```python
from build123d import *

# Parameters (mm, degrees)
F1_W     = 59.7976446152
F1_H     = 97.4377058446
F1_R     = 17.5
F2_DEPTH = 25
F3_W     = 39.5896174014
F3_H     = 18.2575397193
F4_DEPTH = 29.972
F5_R     = 5.08


with BuildPart() as f2:
    # F1 (on face) → F2 (new body)
    with BuildSketch(Plane.XY):
        with Locations((0, 18.7598057091)):
            Rectangle(F1_W, F1_H)
        Circle(F1_R, mode=Mode.SUBTRACT)
    extrude(amount=F2_DEPTH)

    # F3 (on face) → F4 (cut)
    with BuildSketch(Plane.XZ.offset(29.9590472132)):
        with Locations((-0.5845595151, 9.1287698597)):
            Rectangle(F3_W, F3_H)
    extrude(amount=-F4_DEPTH, mode=Mode.SUBTRACT)

    # F5
    f5_edges = [f2.edges().sort_by_distance(p)[0] for p in [
        (0, -29.959047, 25),
        (29.898822, 18.759806, 25),
        (0, 67.478659, 25),
        (-29.898822, 18.759806, 25),
        (-17.5, 0, 25),
    ]]
    fillet(f5_edges, radius=F5_R)


solid = f2.part
```
Here's how the part is built. I have some questions about the finished solid (model axes, mm). A direction names the side the tool comes from. Coordinates: 2 decimals unless noted, no trailing zeros. Order: outer loops, then holes, each group sorted by start corner. A loop starts at its lowest first (then second) coordinate and runs counter-clockwise, first axis right, second up.
1) Will these pins go through, and if not, where does the flat tip stop? pin 1 (2 mm diameter, centred on x = 5, y = 19.5, fed in from +Z); pin 2 (0.9 mm diameter, centred on x = 18.5, z = 11.5, fed in from -Y).
2) Imagine slicing it at B-B on z = 7. List the corners of the cut face in (x, y) for me, and give its area (3 significant figures).
3) Imagine slicing it at A-A on x = 0. List the corners of the cut face in (y, z) for me.
4) We'd pull the mould along X, two halves only. Please class faces 1 (the face through (-19, 0.013, 9)), 2 (the face through (-1, -19, 18.258)), 3 (the face through (28.37, 19.44, 23.55)), 4 (the face through (0, 30, 0)): +X half, -X half, draft (parallel to the pull), parting line (faces both ways), or undercut.
5) Which directions (+Z, -Z, +X, -X, +Y, -Y) give clear straight access to the entire face, cutting with the end or side of a thin tool? Please do faces 5 (the face through (29.899, 18, 10)), 6 (the face through (-20.379, -15, 9)).
6) I need wall thicknesses on line 1 (X direction, y = -18, z = 10.5); line 2 (Y direction, x = 0, z = 15.5); line 3 (X direction, y = 7, z = 4.5). Which ranges of each line are inside material? Lowest first, please.
Response values:
1. pin 1: stops at z = 24.79
1. pin 2: stops at y = 0.01
2. outline: (-29.9, -29.96) - (-20.38, -29.96) - (-20.38, 0.01) - (-17.5, 0.01) arc R17.5 cw to (17.5, 0.01) - (19.21, 0.01) - (19.21, -29.96) - (29.9, -29.96) - (29.9, 67.48) - (-29.9, 67.48) - close
2. area: 4,160 mm2
3. outline: (-29.96, 18.26) - (-17.5, 18.26) - (-17.5, 19.92) arc R5.08 ccw to (-22.58, 25) - (-24.88, 25) arc R5.08 ccw to (-29.96, 19.92) - close; (17.5, 0) - (67.48, 0) - (67.48, 19.92) arc R5.08 ccw to (62.4, 25) - (22.58, 25) arc R5.08 ccw to (17.5, 19.92) - close
4. face 1: undercut
4. face 2: undercut
4. face 3: +X half
4. face 4: draft
5. face 5: +Z, -Z, +X, +Y, -Y
5. face 6: -Z, -Y
6. line 1: x = -29.9 to -20.38, 19.21 to 29.9
6. line 2: y = 17.5 to 67.48
6. line 3: x = -29.9 to -16.04, 16.04 to 29.9
